from build123d import *

# Parameters (mm, degrees)
SKETCH_1_R      = 1.15
EXTRUDE_1_DEPTH = 2
FILLET_1_R      = 6.5


with BuildPart() as part:
    # Эскиз1 → Бобышка-Вытянуть1 (new body)
    with BuildSketch(Plane(origin=(0, 0, 0), x_dir=(1, 0, 0), z_dir=(0, 1, 0))):
        with BuildLine():
            Line((2.236067977, 2), (17.463932023, 2))
            ThreePointArc((17.463932023, 2), (22.7, 0), (17.463932023, -2))
            Line((17.463932023, -2), (2.236067977, -2))
            ThreePointArc((2.236067977, -2), (-3, 0), (2.236067977, 2))
        make_face()
        with Locations(Location((0, 0, 0), (0, 0, 270))):
            Circle(SKETCH_1_R, mode=Mode.SUBTRACT)
        with Locations(Location((19.7, 0, 0), (0, 0, 270))):
            Circle(SKETCH_1_R, mode=Mode.SUBTRACT)
    extrude(amount=EXTRUDE_1_DEPTH)

    # Скругление1
    fillet_1_edges = [part.edges().sort_by_distance(p)[0] for p in [
        (2.236067977, 1, 2),
        (2.236067977, 1, -2),
        (17.463932023, 1, -2),
        (17.463932023, 1, 2),
    ]]
    fillet(fillet_1_edges, radius=FILLET_1_R)


solid = part.part
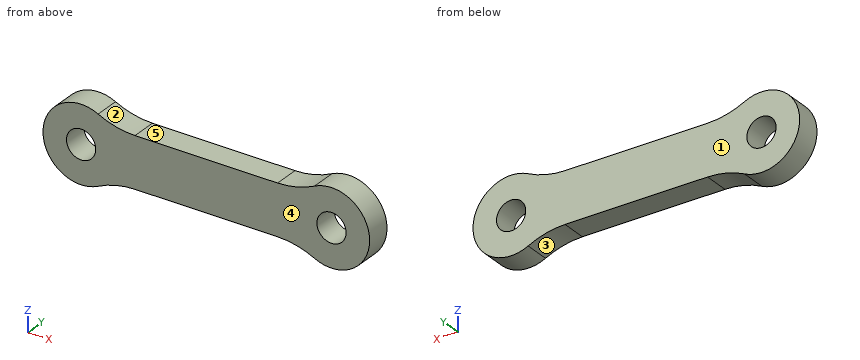
Part model, mm, in its own coordinate system. Face numbers are marked on the shaded views. A direction names the side the tool comes from. Coordinates: 2 decimals unless noted, no trailing zeros. Loops run counter-clockwise (first coordinate to the right, second up) from the corner with the lowest first, then second, coordinate; pieces in that order, holes last. Notation, with made-up numbers: (16, -6.5) - (39, -6.5) arc R19 ccw to (39, 16.5) - close; hole circle Ø4 at (75, 81.25). An arc over 180 degrees is marked (long way). Write each question's results on one line, items separated by ' | '. Start each with the question number.
Q1. Drop flat-ended pins along their axis: pin 1 Ø0.6 at (x, y) = (7.5, 1) entering from +Z; pin 2 Ø2.5 at (x, z) = (0, 0) entering from +Y; pin 3 Ø2 at (x, z) = (19.7, 0) entering from +Y; pin 4 Ø1 at (x, y) = (8, 1) entering from -Z. Give the stop position or say it passes through.
Q2. Slice it at D-D on x = 19.25. Give the cut face in (y, z).
Q3. Probe line 1 along Z through (x, y) = (9.5, 0.25); line 2 along X through (y, z) = (0.9, 0.9); line 3 along X through (y, z) = (0.6, 0.5). List the from-to ranges inside material, lowest first.
Q4. Which spindle directions (+Z, -Z, +X, -X, +Y, -Y) get a long thin tool onto all of the face, cutting with end or side? Do the marked faces 3, 4 and 5. Say none if no direction does.
Q5. Slice it at B-B on y = 1.35. Give the cut face in (x, z).
Q6. Two-plate mould, pull along X, no slides. Class the marked faces 1 and 2: +X half, -X half, draft (parallel to the pull), parting line (faces both ways), or undercut.
Q7. Slice it at A-A on z = 0. Give the cut face in (x, y).
Q8. Slice it at C-C on x = 0. Give the cut face in (y, z).
Answer:
1) pin 1: stops at z = 2 | pin 2: stops at y = 2 | pin 3: passes through | pin 4: stops at z = -2
2) outline: (0, -2.97) - (2, -2.97) - (2, -1.06) - (0, -1.06) - close; (0, 1.06) - (2, 1.06) - (2, 2.97) - (0, 2.97) - close
3) line 1: z = -2 to 2 | line 2: x = -2.86 to -0.72, 0.72 to 18.98, 20.42 to 22.56 | line 3: x = -2.96 to -1.04, 1.04 to 18.66, 20.74 to 22.66
4) face 3: -Z, +Y, -Y | face 4: +Z, -Z, +X, -X, -Y | face 5: +Z, +Y, -Y
5) outline: (1.34, -2.68) arc R6.5 cw to (4.24, -2) - (15.46, -2) arc R6.5 cw to (18.36, -2.68) arc R3 ccw (long way) to (18.36, 2.68) arc R6.5 cw to (15.46, 2) - (4.24, 2) arc R6.5 cw to (1.34, 2.68) arc R3 ccw (long way) to start; hole circle Ø2.3 at (0, 0); hole circle Ø2.3 at (19.7, 0)
6) face 1: draft | face 2: undercut
7) outline: (-3, 0) - (-1.15, 0) - (-1.15, 2) - (-3, 2) - close; (1.15, 0) - (18.55, 0) - (18.55, 2) - (1.15, 2) - close; (20.85, 0) - (22.7, 0) - (22.7, 2) - (20.85, 2) - close
8) outline: (0, -3) - (2, -3) - (2, -1.15) - (0, -1.15) - close; (0, 1.15) - (2, 1.15) - (2, 3) - (0, 3) - close
